from build123d import *

# Parameters (mm, degrees)
BOSS_EXTRUDE1_DEPTH = 50
BOSS_EXTRUDE2_DEPTH = 16.5
CUT_EXTRUDE1_DEPTH  = 16.5
CUT_EXTRUDE2_REACH  = 141.217
FILLET1_R           = 10


with BuildPart() as part:
    # Sketch1 → Boss-Extrude1 (new body)
    with BuildSketch(Plane.XY):
        Polygon((54.481827389, 0), (0, 0), (-51.739424843, -53.577742843), (-61.090842247, -44.547184027), (-5.518172611, 13), (54.481827389, 13), align=None)
    extrude(amount=BOSS_EXTRUDE1_DEPTH)

    # Sketch4 → Boss-Extrude2 (add, symmetric)
    with BuildSketch(Plane(origin=(-4.675708702, 4.515279408, 0), x_dir=(0, 0, -1), z_dir=(0.7193398003386524, -0.6946583704589959, 0))):
        with BuildLine():
            Line((-50, -54.481827389), (0, -54.481827389))
            ThreePointArc((0, -54.481827389), (20, -74.481827389), (0, -94.481827389))
            Line((0, -94.481827389), (-50, -94.481827389))
            ThreePointArc((-50, -94.481827389), (-70, -74.481827389), (-50, -54.481827389))
        make_face()
        with BuildLine():
            Line((-50, -65.481827389), (0, -65.481827389))
            ThreePointArc((0, -65.481827389), (9, -74.481827389), (0, -83.481827389))
            Line((0, -83.481827389), (-50, -83.481827389))
            ThreePointArc((-50, -83.481827389), (-59, -74.481827389), (-50, -65.481827389))
        make_face(mode=Mode.SUBTRACT)
    extrude(amount=BOSS_EXTRUDE2_DEPTH, both=True)

    # Sketch4<2> → Cut-Extrude1 (cut, symmetric)
    with BuildSketch(Plane(origin=(-4.675708702, 4.515279408, 0), x_dir=(0, 0, -1), z_dir=(0.7193398003386524, -0.6946583704589959, 0))):
        with BuildLine():
            Line((-50, -83.481827389), (0, -83.481827389))
            ThreePointArc((0, -83.481827389), (9, -74.481827389), (0, -65.481827389))
            Line((0, -65.481827389), (-50, -65.481827389))
            ThreePointArc((-50, -65.481827389), (-59, -74.481827389), (-50, -83.481827389))
        make_face()
    extrude(amount=CUT_EXTRUDE1_DEPTH, both=True, mode=Mode.SUBTRACT)

    # Sketch6 → Cut-Extrude2 (cut, up to next)
    with BuildSketch(Plane(origin=(0, 13, 0), x_dir=(1, 0, 0), z_dir=(0, 1, 0)), mode=Mode.PRIVATE) as cut_extrude2_sk1:
        with BuildLine():
            Line((19.481827389, -12.5), (54.481827389, -12.5))
            ThreePointArc((54.481827389, -12.5), (66.981827389, -25), (54.481827389, -37.5))
            Line((54.481827389, -37.5), (19.481827389, -37.5))
            ThreePointArc((19.481827389, -37.5), (6.981827389, -25), (19.481827389, -12.5))
        make_face()
    cut_extrude2_tool1 = extrude(cut_extrude2_sk1.sketch, amount=-CUT_EXTRUDE2_REACH, mode=Mode.PRIVATE) & part.part
    add(cut_extrude2_tool1.solids().sort_by_distance((36.981827, 13, 25))[0], mode=Mode.SUBTRACT)

    # Fillet1
    fillet1_edges = [part.edges().sort_by_distance(p)[0] for p in [
        (54.481827389, 6.5, 50),
        (54.481827389, 6.5, 0),
    ]]
    fillet(fillet1_edges, radius=FILLET1_R)


solid = part.part
Geometry check sheet. Reference: the model listing, model coordinates, mm. A direction names the side the tool comes from. Round coordinates to 2 decimals unless told otherwise and drop trailing zeros. Order: outer loops, then holes, each group sorted by start corner. A loop starts at its lowest first (then second) coordinate and runs counter-clockwise, first axis right, second up. Notation, with made-up numbers: M -6,66.5 L 39,66.5 A24 cw 39,94.5 Z; hole C -6.5,-5.5 d6. An arc over 180 degrees is marked long. Answer in a Markdown table with one row per item. Add a question column.
Item 1: Set-up check for faces 1 (the face through (22, 0, 41)), 2 (the face through (-50.74, -26.74, 25.35)), 3 (the face through (-34.2, -42.71, 25.35)), 4 (the face through (-56.111, -49.081, -8.998)), 5 (the face through (-5, -1, 0)): record each of +Z, -Z, +X, -X, +Y, -Y from which the full face is reachable in a straight line by a thin tool's end or side.
Item 2: Sectioned sample at D-D, the plane z = 2. Enter the section's corners in (x, y), plus the area to 3 significant figures.
Item 3: Sectioned sample at A-A, the plane z = 25. Enter the section's corners in (x, y).
Item 4: Sectioned sample at B-B, the plane x = 37. Enter the section's corners in (y, z).
Item 5: Draft check along Z on faces 6 (the face through (51.475, 6.409, 2.852)), 7 (the face through (-61.915, -31.005, 24.37)), 8 (the face through (-49.997, -42.749, 25.35)). Enter one of: released by +Z, released by -Z, zero draft, split by the parting line, or undercut.
Item 6: Depth check by flat-ended pin: pin 1 Ø6 at (x, z) = (-67.5, 11.5) entering from +Y; pin 2 Ø2 at (y, z) = (-27.5, 22) entering from +X; pin 3 Ø15.5 at (x, y) = (-12.5, -17.5) entering from -Z; pin 4 Ø4 at (x, z) = (30, 15.5) entering from +Y. Enter the tip coordinate at first touch or a pass-through.
Item 7: Sectioned sample at C-C, the plane x = 14. Enter the section's corners in (y, z), plus the area to 3 significant figures.
Item 8: Material ranges on L1, parallel to Y at x = -35, z = 2.5; L2, parallel to Y at x = -32, z = 25.5; L3, parallel to X at y = -28.5, z = 27.5, recorded low to high. Write a range as [from, to].
Filled in:
| question | item | result |
|---|---|---|
| 1 | face 1 | +Z, -Z, +X, -Y |
| 1 | face 2 | +Z, -Z, +Y |
| 1 | face 3 | +Z, -Z, +X |
| 1 | face 4 | none |
| 1 | face 5 | -Z, +X, +Y |
| 2 | outline | M -82.18,-51.99 L -58.44,-74.91 L -50.8,-67 L -74.54,-44.07 Z; M -62.03,-31.13 L -38.29,-54.05 L -30.65,-46.14 L -37.85,-39.19 L 0,0 L 50.48,0 L 50.48,13 L -5.52,13 L -47.2,-30.16 L -54.39,-23.21 Z |
| 2 | area | 2,160 mm² |
| 3 | outline | M -82.18,-51.99 L -58.44,-74.91 L -50.8,-67 L -74.54,-44.07 Z; M -62.03,-31.13 L -38.29,-54.05 L -30.65,-46.14 L -37.85,-39.19 L 0,0 L 6.98,0 L 6.98,13 L -5.52,13 L -47.2,-30.16 L -54.39,-23.21 Z |
| 4 | outline | M 0,0 L 13,0 L 13,12.5 L 0,12.5 Z; M 0,37.5 L 13,37.5 L 13,50 L 0,50 Z |
| 5 | face 6 | released by -Z |
| 5 | face 7 | zero draft |
| 5 | face 8 | undercut |
| 6 | pin 1 | stops at y = -47.97 |
| 6 | pin 2 | stops at x = -25.59 |
| 6 | pin 3 | stops at z = 0 |
| 6 | pin 4 | passes through |
| 7 | outline | M 0,0 L 13,0 L 13,13.77 L 0,13.77 Z; M 0,36.23 L 13,36.23 L 13,50 L 0,50 Z |
| 7 | area | 358 mm² |
| 8 | L1 | y = [-50.64, -41.94], [-36.24, -17.53] |
| 8 | L2 | y = [-47.53, -44.84], [-33.14, -14.42] |
| 8 | L3 | x = [-59.5, -48.92], [-45.59, -27.52] |
